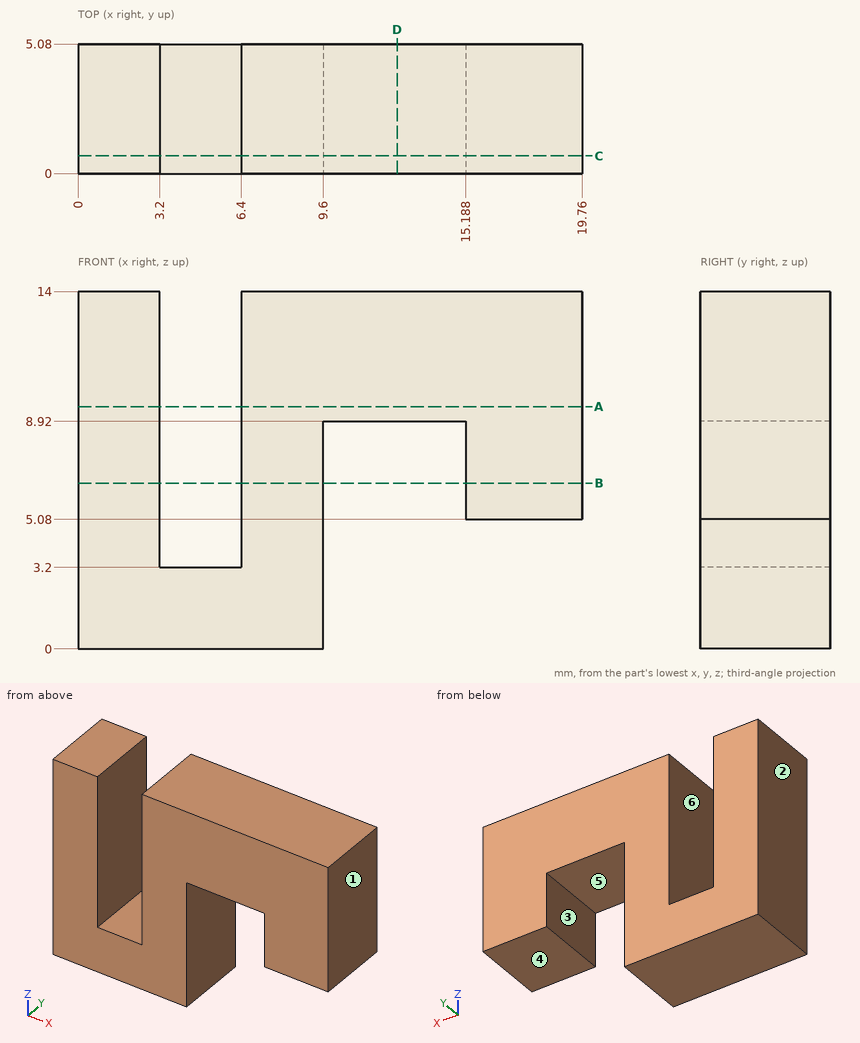
Here's the drawing with two shaded views (mm, measured from the low corner). I have some questions. A direction names the side the tool comes from. Give positions to 0.01 mm unless a question says otherwise; leave off trailing zeros. Loops run counter-clockwise (first coordinate to the right, second up) from the corner with the lowest first, then second, coordinate; pieces in that order, holes last. Notation, with made-up numbers: (-19, 62.5) -> (37, 62.5) arc R16 ccw to (37, 79.5) -> close; hole circle Ø10 at (76.5, 66). An arc over 180 degrees is marked (long way). Use one line per item in the form item = value.
1) If we section it at C-C (y = 0.7): Please give me the cut outline in (x, z), plus the area to 3 significant figures.
Answers:
outline = (0, 0) -> (9.6, 0) -> (9.6, 8.92) -> (15.19, 8.92) -> (15.19, 5.08) -> (19.76, 5.08) -> (19.76, 14) -> (6.4, 14) -> (6.4, 3.2) -> (3.2, 3.2) -> (3.2, 14) -> (0, 14) -> close
area = 169 mm²
2) Will these pins go through, and if not, where does the flat tip stop? pin 1 (1.5 mm diameter, centred on x = 11.5, y = 2, fed in from -Z); pin 2 (1.5 mm diameter, centred on y = 2.5, z = 4, fed in from +X); pin 3 (1.4 mm diameter, centred on x = 16.5, y = 1.5, fed in from -Z).
Answers:
pin_1 = 8.92
pin_2 = 9.6
pin_3 = 5.08
3) If we section it at D-D (x = 12.5): Please give me the cut outline in (y, z).
Answers:
outline = (0, 8.92) -> (5.08, 8.92) -> (5.08, 14) -> (0, 14) -> close
4) I need wall thicknesses on line 1 along X through (y, z) = (1.35, 8); line 2 along X through (y, z) = (2.2, 9.75); line 3 along X through (y, z) = (3.25, 3.25). Which ranges of each line are inside material? Lowest first, please.
Answers:
line_1 = 0 to 3.2, 6.4 to 9.6, 15.19 to 19.76
line_2 = 0 to 3.2, 6.4 to 19.76
line_3 = 0 to 3.2, 6.4 to 9.6
5) For the marked faces 4, 5 and 6, which set-ups out of +Z, -Z, +X, -X, +Y, -Y let a thin tool reach every point of the face, with its end or its side?
Answers:
face_4 = -Z, +X, +Y, -Y
face_5 = -Z, +Y, -Y
face_6 = +Z, +Y, -Y
6) If we section it at B-B (z = 6.5): Please give me the cut outline in (x, y), plus the area to 3 significant figures.
Answers:
outline = (0, 0) -> (3.2, 0) -> (3.2, 5.08) -> (0, 5.08) -> close; (6.4, 0) -> (9.6, 0) -> (9.6, 5.08) -> (6.4, 5.08) -> close; (15.19, 0) -> (19.76, 0) -> (19.76, 5.08) -> (15.19, 5.08) -> close
area = 55.7 mm²
7) If we section it at A-A (z = 9.5): Please give me the cut outline in (x, y), plus the area to 3 significant figures.
Answers:
outline = (0, 0) -> (3.2, 0) -> (3.2, 5.08) -> (0, 5.08) -> close; (6.4, 0) -> (19.76, 0) -> (19.76, 5.08) -> (6.4, 5.08) -> close
area = 84.1 mm²
8) We'd pull the mould along X, two halves only. Please class the marked faces 1, 2 and 3: released by +X, released by -X, zero draft, split by the parting line, or undercut.
Answers:
face_1 = released by +X
face_2 = released by -X
face_3 = undercut
